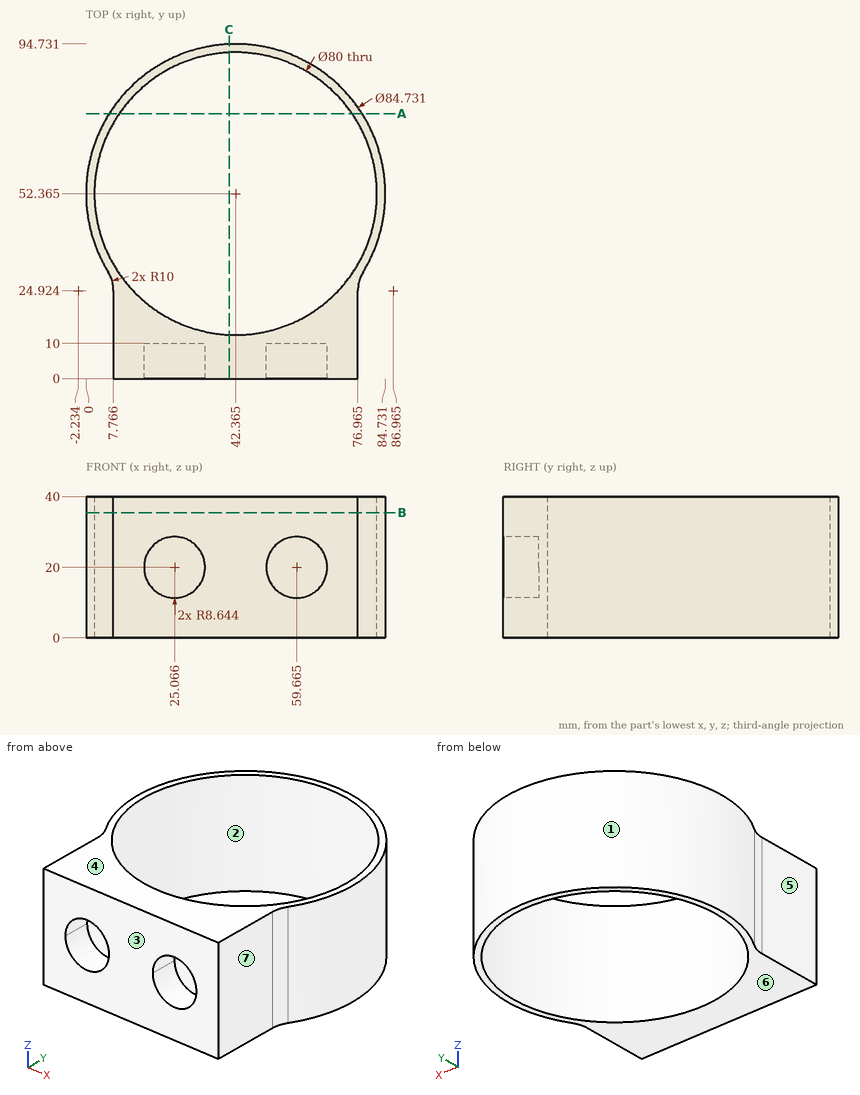
Drawing for the job (mm, zero at the part's lowest x, y, z). A direction names the side the tool comes from. Coordinates: 2 decimals unless noted, no trailing zeros. Loops run counter-clockwise (first coordinate to the right, second up) from the corner with the lowest first, then second, coordinate; pieces in that order, holes last. Notation, with made-up numbers: (-33.75, -27.5) - (16.25, -27.5) arc R26 ccw to (16.25, -1.5) - close; hole circle Ø1 at (10, 20). An arc over 180 degrees is marked (long way). Return JSON: item names as keys, results as strings.
1. Probe L1, parallel to X at y = 71, z = 5; L2, parallel to X at y = 39, z = 5 (1 decimal); L3, parallel to Y at x = 20.5, z = 7. List the from-to ranges inside material, lowest first. Write a range as from..to.
Result:
{"L1": "x = 4.32..6.97, 77.76..80.41", "L2": "x = 2.2..4.7, 80.1..82.6", "L3": "y = 0..18.87, 85.86..88.65"}
2. Drop flat-ended pins along their axis: pin 1 (12.5 mm diameter, centred on y = 8.5, z = 29, fed in from +X) (1 decimal); pin 2 (3 mm diameter, centred on x = 52.5, z = 17, fed in from +Y); pin 3 (5 mm diameter, centred on x = 55.5, z = 16, fed in from -Y). Give the stop position or say it passes through.
Result:
{"pin 1": "stops at x = 77", "pin 2": "stops at y = 93.84", "pin 3": "stops at y = 10"}
3. Band-saw the part on A-A (y = 75). Give the cut face in (x, z) (1 decimal).
Result:
{"outline": "(6.6, 0) - (9.4, 0) - (9.4, 40) - (6.6, 40) - close; (75.3, 0) - (78.2, 0) - (78.2, 40) - (75.3, 40) - close"}
4. Band-saw the part on B-B (z = 35.5). Give the cut face in (x, y) (1 decimal).
Result:
{"outline": "(6.3, 30.2) arc R10 cw to (7.8, 24.9) - (7.8, 0) - (77, 0) - (77, 24.9) arc R10 cw to (78.4, 30.2) arc R42.4 ccw (long way) to start; hole circle Ø80 at (42.4, 52.4)"}
5. Mould opens along Y. For the marked faces 1, 2, 3 and 4 say: released by +Y, released by -Y, zero draft, split by the parting line, or undercut.
Result:
{"face 1": "split by the parting line", "face 2": "undercut", "face 3": "released by -Y", "face 4": "zero draft"}
6. 3-axis set-ups, long thin cutter, end or side, ignore diameter. For the marked faces 5, 6 and 7: which of +Z, -Z, +X, -X, +Y, -Y reach the whole face in a straight line?
Result:
{"face 5": "+Z, -Z, -X, -Y", "face 6": "-Z, +X, -X, +Y, -Y", "face 7": "+Z, -Z, +X, -Y"}
7. Band-saw the part on C-C (x = 40.5). Give the cut face in (y, z), and give its area (3 significant figures).
Result:
{"outline": "(0, 0) - (12.41, 0) - (12.41, 40) - (0, 40) - close; (92.32, 0) - (94.69, 0) - (94.69, 40) - (92.32, 40) - close", "area": "591 mm2"}
